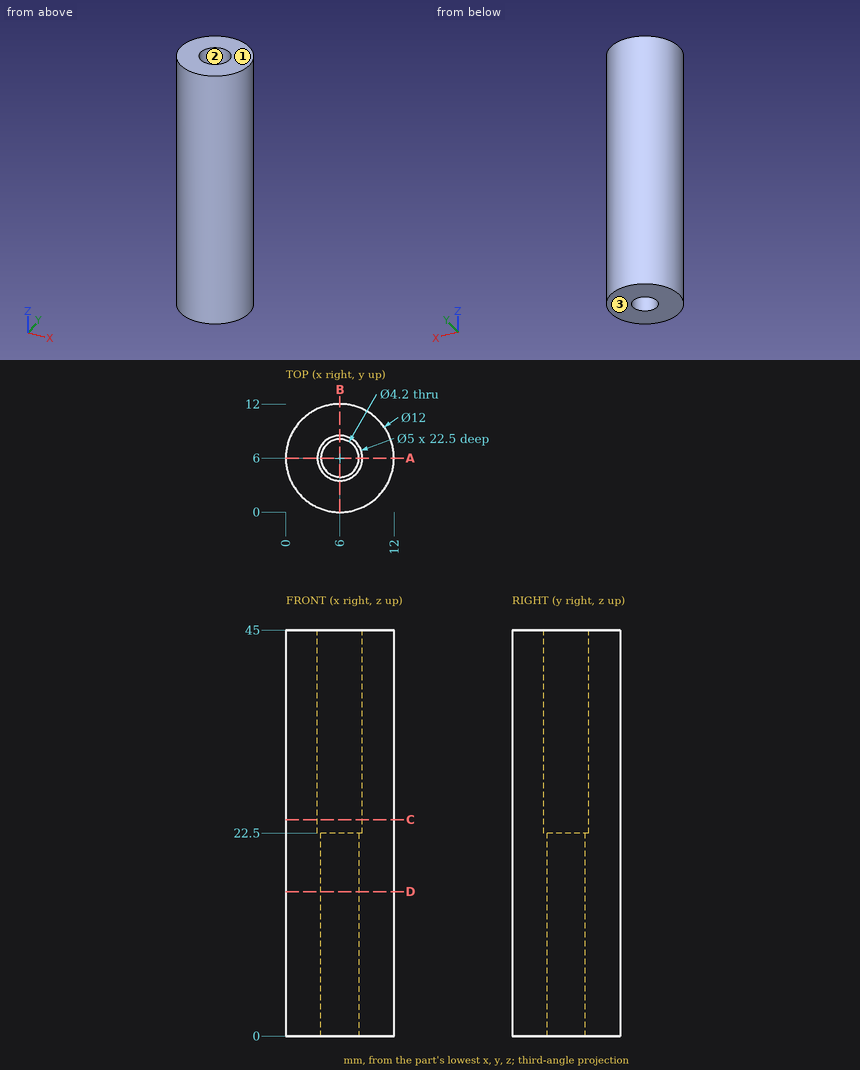
The drawing under review shows one solid part. Ordinate dimensions are in mm from its lowest x, y, z. Round coordinates to 2 decimals unless told otherwise and drop trailing zeros. Order: outer loops, then holes, each group sorted by start corner. A loop starts at its lowest first (then second) coordinate and runs counter-clockwise, first axis right, second up. Notation, with made-up numbers: (21.5, 3) -> (67.5, 3) arc R17 ccw to (67.5, 30) -> close; hole circle Ø8 at (21.25, 15.25). An arc over 180 degrees is marked (long way). Use a Markdown table: item, result.
Item 1: For line 1 along Y through (x, z) = (6, 12.5); line 2 along Y through (x, z) = (6, 27.5); line 3 along Z through (x, y) = (4.25, 7.75), list the stretches that pass through material, from the lowest coordinate up. Write a range as [from, to].
Resolved:
| item | result |
|---|---|
| line 1 | y = [0, 3.9], [8.1, 12] |
| line 2 | y = [0, 3.5], [8.5, 12] |
| line 3 | z = [0, 22.5] |
Item 2: Take a section at A-A (y = 6). State the section outline as (x, z) points, plus the area to 3 significant figures.
Resolved:
| item | result |
|---|---|
| outline | (0, 0) -> (3.9, 0) -> (3.9, 22.5) -> (3.5, 22.5) -> (3.5, 45) -> (0, 45) -> close; (8.1, 0) -> (12, 0) -> (12, 45) -> (8.5, 45) -> (8.5, 22.5) -> (8.1, 22.5) -> close |
| area | 333 mm² |
Item 3: For pin 1 (1.5 mm diameter, centred on x = 10, z = 39, fed in from -Y); pin 2 (3 mm diameter, centred on x = 9.5, z = 8, fed in from +Y); pin 3 (5 mm diameter, centred on x = 2, z = 10.5, fed in from +Y), all flat-tipped, find the tip position at first contact; note any pin that passes through.
Resolved:
| item | result |
|---|---|
| pin 1 | stops at y = 0.96 |
| pin 2 | stops at y = 11.66 |
| pin 3 | stops at y = 11.81 |
Item 4: Take a section at D-D (z = 16). State the section outline as (x, y) points.
Resolved:
| item | result |
|---|---|
| outline | circle Ø12 at (6, 6); hole circle Ø4.2 at (6, 6) |
Item 5: Take a section at C-C (z = 24). State the section outline as (x, y) points, plus the area to 3 significant figures.
Resolved:
| item | result |
|---|---|
| outline | circle Ø12 at (6, 6); hole circle Ø5 at (6, 6) |
| area | 93.5 mm² |
Item 6: Draft analysis for pull direction Z (two halves, no side actions). For the marked faces 1, 2 and 3, state which applies: +Z half, -Z half, draft (parallel to the pull), parting line (faces both ways), or undercut.
Resolved:
| item | result |
|---|---|
| face 1 | +Z half |
| face 2 | draft |
| face 3 | -Z half |
